The model under review builds one solid part; all positions refer to its coordinate system, in mm. A direction names the side the tool comes from. Round coordinates to 2 decimals unless told otherwise and drop trailing zeros. Order: outer loops, then holes, each group sorted by start corner. A loop starts at its lowest first (then second) coordinate and runs counter-clockwise, first axis right, second up.
```python
from build123d import *

# Parameters (mm, degrees)
BOSS_EXTRUDE1_DEPTH = 10.033
SKETCH2_R           = 3.048
SKETCH2_R_2         = 2.54
CUT_EXTRUDE1_DEPTH  = 10.033
SKETCH3_R           = 2.286
CUT_EXTRUDE2_DEPTH  = 10.033


with BuildPart() as part:
    # Sketch1 → Boss-Extrude1 (new body, symmetric)
    with BuildSketch(Plane(origin=(0, 0, 0), x_dir=(1, 0, 0), z_dir=(0, 1, 0))):
        with BuildLine():
            Line((24.384, -12.319), (24.384, 12.319))
            Line((24.384, 12.319), (3.973043901, 17.069727536))
            ThreePointArc((3.973043901, 17.069727536), (-9.658201012, 14.624630908), (-17.258921519, 3.048))
            Line((-17.258921519, 3.048), (-43.942, 3.048))
            Line((-43.942, 3.048), (-43.942, -3.048))
            Line((-43.942, -3.048), (-17.258921519, -3.048))
            ThreePointArc((-17.258921519, -3.048), (-9.658201012, -14.624630908), (3.973043901, -17.069727536))
            Line((3.973043901, -17.069727536), (24.384, -12.319))
        make_face()
        with BuildLine():
            Line((21.336, -9.898960775), (21.336, 9.898960775))
            Line((21.336, 9.898960775), (3.282079744, 14.101079269))
            ThreePointArc((3.282079744, 14.101079269), (-14.478, 0), (3.282079744, -14.101079269))
            Line((3.282079744, -14.101079269), (21.336, -9.898960775))
        make_face(mode=Mode.SUBTRACT)
    extrude(amount=BOSS_EXTRUDE1_DEPTH, both=True)

    # Sketch2 → Cut-Extrude1 (cut, symmetric)
    with BuildSketch(Plane.XY.offset(3.048)):
        with Locations((-37.846, 0)):
            Circle(SKETCH2_R)
        with Locations((-22.606, 0)):
            Circle(SKETCH2_R_2)
    extrude(amount=CUT_EXTRUDE1_DEPTH, both=True, mode=Mode.SUBTRACT)

    # Sketch3 → Cut-Extrude2 (cut, symmetric)
    with BuildSketch(Plane(origin=(24.384, 0, 0), x_dir=(0, 0, -1), z_dir=(1, 0, 0))):
        Circle(SKETCH3_R)
    extrude(amount=CUT_EXTRUDE2_DEPTH, both=True, mode=Mode.SUBTRACT)


solid = part.part
```
(1) Consider section D-D (y = 0). Write out the cut boundary in (x, z).
Data:
outline: (-43.94, -3.05) - (-40.89, -3.05) - (-40.89, 3.05) - (-43.94, 3.05) - close; (-34.8, -3.05) - (-25.15, -3.05) - (-25.15, 3.05) - (-34.8, 3.05) - close; (-20.07, -3.05) - (-17.26, -3.05) arc R17.53 ccw to (3.97, -17.07) - (24.38, -12.32) - (24.38, -2.29) - (21.34, -2.29) - (21.34, -9.9) - (3.28, -14.1) arc R14.48 cw (long way) to (3.28, 14.1) - (21.34, 9.9) - (21.34, 2.29) - (24.38, 2.29) - (24.38, 12.32) - (3.97, 17.07) arc R17.53 ccw to (-17.26, 3.05) - (-20.07, 3.05) - close
(2) For faces 5 (the flat face through (12.18, 0.14, 12.03)), 6 (the flat face through (14.32, 0.14, -14.66)), 7 (the flat face through (-31, 0, 3.048)), 8 (the cylindrical face through (22.88, -2.23, 0.5)), 9 (the cylindrical face through (-20.26, -0.97, 0.04)), list the 3-axis set-ups (+Z, -Z, +X, -X, +Y, -Y) from which the entire face can be reached by the end or side of a thin tool; tool diameter is ignored.
Data:
face 5: +Y, -Y
face 6: -Z, +X, +Y, -Y
face 7: +Z, -X, +Y, -Y
face 8: +X
face 9: +Z, -Z
(3) Insertion check: pin 1 (8 mm diameter, centred on x = -37.846, y = 0, fed in from -Z); pin 2 (3 mm diameter, centred on x = -35.5, y = -1.5, fed in from +Z); pin 3 (3 mm diameter, centred on x = -22.606, y = 0, fed in from -Z); pin 4 (6 mm diameter, centred on y = 3.5, z = -6, fed in from -X). Each pin has a flat end and moves straight along its axis. Give the tip position at first contact, or say it passes through.
Data:
pin 1: stops at z = -3.05
pin 2: stops at z = 3.05
pin 3: passes through
pin 4: stops at x = -43.94
(4) To check wall thickness, follow probe 1 along Y at (x, z) = (23.7, 0); probe 2 along Z at (x, y) = (0, -0.5); probe 3 along Z at (x, y) = (-23, -8.75). State the ranges of each line that lie inside material, in increasing order.
Data:
probe 1: y = -10.03 to -2.29, 2.29 to 10.03
probe 2: z = -17.53 to -14.48, 14.48 to 17.53
probe 3: z = -3.05 to 3.05
(5) Draft analysis for pull direction X (two halves, no side actions). For faces 1 (the flat face through (-30, 0, -3.048)), 2 (the flat face through (-43.942, 0, 0)), 3 (the flat face through (21.336, 2, 2)), 4 (the flat face through (12.44, 0.14, -11.97)), state which applies: pulls with the +X half, pulls with the -X half, needs draft (parallel to the pull), parting line crosses it, or undercut.
Data:
face 1: needs draft
face 2: pulls with the -X half
face 3: undercut
face 4: undercut
(6) Consider section B-B (y = 5). Write out the cut boundary in (x, z).
Data:
outline: (-43.94, -3.05) - (-17.26, -3.05) arc R17.53 ccw to (3.97, -17.07) - (24.38, -12.32) - (24.38, 12.32) - (3.97, 17.07) arc R17.53 ccw to (-17.26, 3.05) - (-43.94, 3.05) - close; hole (3.28, -14.1) - (21.34, -9.9) - (21.34, 9.9) - (3.28, 14.1) arc R14.48 ccw (long way) to start
(7) Consider section C-C (x = 0). Write out the cut boundary in (y, z).
Data:
outline: (-10.03, -17.53) - (10.03, -17.53) - (10.03, -14.48) - (-10.03, -14.48) - close; (-10.03, 14.48) - (10.03, 14.48) - (10.03, 17.53) - (-10.03, 17.53) - close
(8) Consider section A-A (z = 0). Write out the cut boundary in (x, y), and give its area (3 significant figures).
Data:
outline: (-43.94, -10.03) - (-14.48, -10.03) - (-14.48, 10.03) - (-43.94, 10.03) - close; (21.34, -10.03) - (24.38, -10.03) - (24.38, -2.29) - (21.34, -2.29) - close; (21.34, 2.29) - (24.38, 2.29) - (24.38, 10.03) - (21.34, 10.03) - close; hole circle Ø6.1 at (-37.85, 0); hole circle Ø5.08 at (-22.61, 0)
area: 589 mm2
